The listing builds one solid part. Answer for the finished solid, in the listing's coordinates (mm). Round coordinates to 2 decimals unless told otherwise and drop trailing zeros. Write each loop counter-clockwise with the first axis right and the second up, starting at its lowest first coordinate (ties: lowest second). Pieces come first, ordered by that corner, then holes.
Autodesk Inventor part; units mm, degrees
ref_plane "YZ Plane" through (0, 0, 0) normal (1, 0, 0) x (0, 1, 0)
ref_plane "XZ Plane" through (0, 0, 0) normal (0, 1, 0) x (-1, 0, 0)
ref_plane "XY Plane" through (0, 0, 0) normal (0, 0, 1) x (1, 0, 0)
sketch "Sketch1" plane through (0, 0, 0) normal (0, 1, 0) x (-1, 0, 0)
  arc A0 (0, -273.05) -> (273.05, 0) centre (0, 0) ccw
  arc A1 (0, -285.75) -> (285.75, 0) centre (0, 0) ccw
  arc A2 (0, -146.05) -> (146.05, 0) centre (0, 0) ccw
  arc A3 (0, -133.35) -> (133.35, 0) centre (0, 0) ccw
  line L0 (0, -285.75) -> (-6.35, -285.75)
  line L1 (146.05, 0) -> (146.05, 6.35)
  line L2 (133.35, 0) -> (133.35, 6.35)
  line L3 (273.05, 6.35) -> (273.05, 0)
  line L4 (285.75, 6.35) -> (285.75, 0)
  circle A4 centre (103.1708, -94.1906) radius 3.3782
  circle A5 centre (94.1906, -103.1708) radius 3.3782
  circle A6 centre (279.4, 0) radius 3.3782
  circle A7 centre (139.7, 0) radius 3.3782
  circle A8 centre (202.0047, -193.0245) radius 3.3782
  circle A9 centre (193.0245, -202.0047) radius 3.3782
  circle A10 centre (0, -279.4) radius 3.3782
  circle A11 centre (0, -139.7) radius 3.3782
  circle A12 centre (-55.2746, -139.7) radius 3.3782
  circle A13 centre (-78.3684, -279.4) radius 3.3782
  line L5 (285.75, 6.35) -> (273.05, 6.35)
  line L6 (146.05, 6.35) -> (133.35, 6.35)
  line L7 (-314.96, -285.75) -> (-314.96, -273.05)
  line L8 (-101.6, -133.35) -> (-127, -133.35)
  line L9 (-127, -146.05) -> (-101.6, -146.05)
  line L10 (-314.96, -146.05) -> (-314.96, -133.35)
  line L11 (-6.35, -285.75) -> (-6.35, -393.7)
  line L12 (-6.35, -393.7) -> (-314.325, -393.7)
  line L13 (-314.325, -393.7) -> (-314.325, -76.2)
  line L14 (-314.325, -76.2) -> (-120.65, -76.2)
  line L15 (-120.65, -76.2) -> (0, -133.35)
  line L16 (0, -285.75) -> (-6.35, -285.75)
  line L17 (0, -146.05) -> (0, -273.05)
  dimension "d10" = 12.7
  dimension "d11" = 12.7
  dimension "d13" = 12.7
  dimension "d14" = 6.7564
  dimension "d15" = 6.7564
  dimension "d16" = 6.7564
  dimension "d18" = 6.7564
  dimension "d20" = 6.35
  dimension "d21" = 6.7564
  dimension "d22" = 6.7564
  dimension "d23" = 6.7564
  dimension "d26" = 6.7564
  dimension "d30" = 6.7564
  dimension "d32" = 6.7564
  dimension "d66" = 25.4
  dimension "d67" = 0
  dimension "d72" = 12.7
  dimension "d81" = 107.95
  dimension "d82" = 133.35
  dimension "d83" = 279.4
  dimension "d84" = 6.35
  dimension "d85" = 317.5
  dimension "d86" = 193.675
  dimension "d87" = 55.2746
  dimension "d88" = 139.7
  dimension "d91" = 307.975
extrude "Extrusion7" add sketch "Sketch1" along normal blind 6.35
sketch "Sketch7" plane through (0, 0, 0) normal (0, -1, 0) x (1, 0, 0)
  line L0 (0, -273.05) -> (0, -146.05)
  line L1 (314.325, -76.2) -> (314.325, -393.7)
  line L2 (314.325, -234.95) -> (0, -234.95)
  line L3 (301.625, -139.7) -> (301.625, -165.1)
  line L4 (301.625, -165.1) -> (98.425, -165.1)
  line L5 (98.425, -165.1) -> (98.425, -139.7)
  line L6 (98.425, -139.7) -> (301.625, -139.7)
  line L7 (301.625, -330.2) -> (301.625, -304.8)
  line L8 (301.625, -304.8) -> (98.425, -304.8)
  line L9 (98.425, -304.8) -> (98.425, -330.2)
  line L10 (98.425, -330.2) -> (301.625, -330.2)
  dimension "d92" = 25.4
  dimension "d93" = 203.2
  dimension "d94" = 12.7
  dimension "d95" = 69.85
extrude "Extrusion8" cut sketch "Sketch7" against normal blind 6.35
sketch "Sketch8" plane through (0, 6.35, 0) normal (0, 1, 0) x (1, 0, 0)
  line L0 (98.425, 165.1) -> (301.625, 165.1)
  line L1 (301.625, 304.8) -> (98.425, 304.8)
  circle A0 centre (78.3684, 279.4) radius 3.3782
  line L2 (314.325, 76.2) -> (314.325, 393.7)
  line L3 (314.325, 393.7) -> (6.35, 393.7)
  line L4 (0, 273.05) -> (0, 146.05)
  line L5 (295.275, 367.3082) -> (295.275, 342.9)
  line L6 (295.275, 342.9) -> (28.575, 342.9)
  line L7 (28.575, 342.9) -> (28.575, 371.475)
  line L8 (28.575, 371.475) -> (295.275, 371.475)
  line L9 (295.275, 371.475) -> (295.275, 367.3082)
  line L10 (295.275, 292.1) -> (28.575, 292.1)
  line L11 (28.575, 292.1) -> (28.575, 263.525)
  line L12 (28.575, 263.525) -> (295.275, 263.525)
  line L13 (295.275, 263.525) -> (295.275, 292.1)
  line L14 (295.275, 250.825) -> (28.575, 250.825)
  line L15 (28.575, 250.825) -> (28.575, 222.25)
  line L16 (28.575, 222.25) -> (295.275, 222.25)
  line L17 (295.275, 222.25) -> (295.275, 250.825)
  line L18 (295.275, 209.55) -> (295.275, 180.975)
  line L19 (295.275, 180.975) -> (28.575, 180.975)
  line L20 (28.575, 180.975) -> (28.575, 209.55)
  line L21 (28.575, 209.55) -> (295.275, 209.55)
  dimension "d100" = 90
  dimension "d101" = 22.225
  dimension "d102" = 19.05
  dimension "d103" = 28.575
  dimension "d104" = 266.7
  dimension "d105" = 28.575
  dimension "d106" = 19.05
  dimension "d107" = 12.7
  dimension "d108" = 266.7
  dimension "d109" = 28.575
  dimension "d110" = 28.575
  dimension "d111" = 12.7
  dimension "d112" = 12.7
  dimension "d113" = 266.7
  dimension "d114" = 19.05
  dimension "d115" = 19.05
extrude "Extrusion9" cut sketch "Sketch8" against normal blind 25.4
sketch "Sketch9" plane through (0, 6.35, 0) normal (0, 1, 0) x (1, 0, 0)
  line L0 (314.325, 76.2) -> (314.325, 393.7)
  line L1 (295.275, 371.475) -> (295.275, 88.9)
  line L2 (295.275, 88.9) -> (288.925, 88.9)
  line L3 (288.925, 88.9) -> (288.925, 381)
  line L4 (288.925, 381) -> (295.275, 381)
  line L5 (295.275, 381) -> (295.275, 371.475)
  dimension "d118" = 282.575
  dimension "d119" = 6.35
  dimension "d120" = 292.1
extrude "Extrusion10" cut sketch "Sketch9" against normal blind 25.4
sketch "Sketch10" plane through (0, 6.35, 0) normal (0, 1, 0) x (1, 0, 0)
  line L0 (120.65, 76.2) -> (314.325, 76.2)
  line L1 (0, 273.05) -> (0, 146.05)
  line L2 (120.65, 76.2) -> (120.65, 63.5)
  line L3 (120.65, 63.5) -> (145.3457, 38.8043)
  line L4 (145.3457, 38.8043) -> (302.8387, 38.8043)
  line L5 (302.8387, 38.8043) -> (302.8387, 76.2)
  dimension "d123" = 12.7
  dimension "d124" = 34.925
  dimension "d125" = 135
extrude "Extrusion11" add sketch "Sketch10" against normal blind 6.35
sketch "Sketch13" plane through (0, 6.35, 0) normal (0, 1, 0) x (1, 0, 0)
  line L0 (288.925, 88.9) -> (288.925, 139.7)
  line L1 (288.925, 139.7) -> (98.425, 139.7)
  line L2 (288.925, 381) -> (295.275, 381)
  line L3 (295.275, 88.9) -> (288.925, 88.9)
  line L4 (145.3457, 38.8043) -> (302.8387, 38.8043)
  line L5 (302.8387, 38.8043) -> (302.8387, 76.2)
  line L6 (0, 273.05) -> (0, 146.05)
  line L7 (98.425, 127) -> (98.425, 101.6)
  line L8 (98.425, 101.6) -> (288.925, 101.6)
  line L9 (98.425, 127) -> (288.925, 127)
  line L10 (288.925, 88.9) -> (288.925, 44.45)
  line L11 (288.925, 44.45) -> (295.275, 44.45)
  line L12 (295.275, 44.45) -> (295.275, 88.9)
  dimension "d135" = 25.4
  dimension "d136" = 336.55
  dimension "d137" = 12.7
extrude "Extrusion13" cut sketch "Sketch13" against normal blind 25.4
sketch "Sketch14" plane through (0, 6.35, 0) normal (0, 1, 0) x (1, 0, 0)
  line L0 (311.15, 79.375) -> (304.8, 79.375)
  line L1 (304.8, 79.375) -> (304.8, 85.725)
  line L2 (304.8, 85.725) -> (311.15, 85.725)
  line L3 (311.15, 85.725) -> (311.15, 79.375)
  line L4 (6.35, 381) -> (301.625, 381)
  line L5 (301.625, 381) -> (301.625, 76.2)
  line L6 (301.625, 76.2) -> (314.325, 76.2)
  line L7 (314.325, 76.2) -> (314.325, 393.7)
  line L8 (314.325, 393.7) -> (6.35, 393.7)
  line L9 (6.35, 393.7) -> (6.35, 381)
  line L10 (311.15, 390.525) -> (311.15, 384.175)
  line L11 (311.15, 384.175) -> (304.8, 384.175)
  line L12 (304.8, 384.175) -> (304.8, 390.525)
  line L13 (304.8, 390.525) -> (311.15, 390.525)
  line L14 (15.875, 384.175) -> (9.525, 384.175)
  line L15 (9.525, 384.175) -> (9.525, 390.525)
  line L16 (9.525, 390.525) -> (15.875, 390.525)
  line L17 (15.875, 390.525) -> (15.875, 384.175)
  line L18 (145.3457, 38.8043) -> (302.8387, 38.8043)
  line L19 (301.625, 139.7) -> (295.275, 139.7)
  line L20 (152.2186, 54.6793) -> (152.2186, 48.3293)
  line L21 (152.2186, 48.3293) -> (158.5686, 48.3293)
  line L22 (158.5686, 48.3293) -> (158.5686, 54.6793)
  line L23 (158.5686, 54.6793) -> (152.2186, 54.6793)
  dimension "d146" = 6.35
  dimension "d148" = 6.35
  dimension "d149" = 9.525
extrude "Extrusion15" cut sketch "Sketch14" against normal blind 25.4 contours L23 L22 L21 L20
sketch "Sketch16" plane through (0, 6.35, 0) normal (0, 1, 0) x (1, 0, 0)
  line L0 (288.925, 165.1) -> (288.925, 180.975)
  line L1 (288.925, 209.55) -> (288.925, 222.25)
  line L2 (288.925, 250.825) -> (288.925, 263.525)
  line L3 (288.925, 292.1) -> (288.925, 304.8)
  line L4 (295.275, 304.8) -> (295.275, 165.1)
  line L5 (295.275, 165.1) -> (301.625, 165.1)
  line L6 (288.925, 165.1) -> (295.275, 165.1)
  line L7 (288.925, 180.975) -> (295.275, 180.975)
  line L8 (288.925, 222.25) -> (295.275, 222.25)
  line L9 (288.925, 209.55) -> (295.275, 209.55)
  line L10 (288.925, 304.8) -> (295.275, 304.8)
  line L11 (288.925, 292.1) -> (295.275, 292.1)
  line L12 (288.925, 263.525) -> (295.275, 263.525)
  line L13 (288.925, 250.825) -> (295.275, 250.825)
extrude "Extrusion16" add sketch "Sketch16" against normal blind 6.35
sketch "Sketch17" plane through (0, 6.35, 0) normal (0, 1, 0) x (1, 0, 0)
  line L0 (288.925, 44.45) -> (288.925, 101.6)
  line L1 (288.925, 101.6) -> (98.425, 101.6)
  line L2 (98.425, 127) -> (288.925, 127)
  line L3 (288.925, 342.9) -> (28.575, 342.9)
  line L4 (28.575, 371.475) -> (288.925, 371.475)
  line L5 (288.925, 127) -> (288.925, 101.6)
  line L6 (276.225, 127) -> (276.225, 101.6)
  line L7 (288.925, 342.9) -> (288.925, 371.475)
  line L8 (276.225, 371.475) -> (276.225, 342.9)
  dimension "d155" = 12.7
  dimension "d156" = 12.7
extrude "Extrusion17" add sketch "Sketch17" against normal blind 6.35
sketch "Sketch18" plane through (0, 6.35, 0) normal (0, 1, 0) x (1, 0, 0)
  line L0 (288.925, 44.45) -> (288.925, 139.7)
  line L1 (295.275, 139.7) -> (295.275, 44.45)
  line L2 (295.275, 44.45) -> (288.925, 44.45)
  line L3 (145.3457, 38.8043) -> (302.8387, 38.8043)
  line L4 (295.275, 70.5543) -> (288.925, 70.5543)
  dimension "d159" = 31.75
extrude "Extrusion18" add sketch "Sketch18" against normal blind 6.35
sketch "Sketch19" plane through (0, 6.35, 0) normal (0, 1, 0) x (1, 0, 0)
  line L0 (314.325, 393.7) -> (6.35, 393.7)
  line L1 (6.35, 393.7) -> (6.35, 285.75)
  circle A0 centre (76.2, 387.35) radius 3.3782
  dimension "d162" = 6.7564
  dimension "d164" = 6.35
  dimension "d165" = 69.85
extrude "Extrusion19" cut sketch "Sketch19" against normal blind 25.4
sketch "Sketch20" plane through (0, 6.35, 0) normal (0, 1, 0) x (1, 0, 0)
  circle A0 centre (95.25, 387.35) radius 3.3782
extrude "Extrusion20" cut sketch "Sketch20" against normal blind 25.4
sketch "Sketch21" plane through (0, 6.35, 0) normal (0, 1, 0) x (1, 0, 0)
  line L0 (158.5686, 54.6793) -> (158.5686, 48.3293)
  line L1 (145.3457, 38.8043) -> (302.8387, 38.8043)
  line L2 (302.8387, 38.8043) -> (302.8387, 76.2)
  circle A0 centre (155.3936, 67.3793) radius 3.3782
  circle A1 centre (267.9137, 67.3793) radius 3.3782
  dimension "d170" = 6.7564
  dimension "d171" = 6.7564
  dimension "d172" = 28.575
  dimension "d173" = 34.925
  dimension "d174" = 28.575
  dimension "d176" = 3.175
extrude "Extrusion21" cut sketch "Sketch21" against normal blind 25.4
sketch "Sketch22" plane through (0, 6.35, 0) normal (0, 1, 0) x (1, 0, 0)
  line L0 (288.925, 330.2) -> (288.925, 381)
  line L1 (288.925, 381) -> (295.275, 381)
  line L2 (295.275, 381) -> (295.275, 330.2)
  line L3 (288.925, 358.775) -> (295.275, 358.775)
  dimension "d179" = 22.225
extrude "Extrusion22" add sketch "Sketch22" against normal blind 6.35
sketch "Sketch23" plane through (0, 6.35, 0) normal (0, 1, 0) x (1, 0, 0)
  line L0 (158.5686, 48.3293) -> (152.2186, 48.3293)
  line L1 (152.2186, 48.3293) -> (152.2186, 54.6793)
  line L2 (152.2186, 54.6793) -> (158.5686, 54.6793)
  line L3 (158.5686, 54.6793) -> (158.5686, 48.3293)
  line L4 (120.65, 63.5) -> (145.3457, 38.8043)
  line L5 (145.3457, 38.8043) -> (302.8387, 38.8043)
  line L6 (302.8387, 38.8043) -> (302.8387, 76.2)
  line L7 (28.575, 371.475) -> (276.225, 371.475)
  line L8 (302.8387, 61.0293) -> (123.1207, 61.0293)
  dimension "d182" = 22.225
extrude "Extrusion23" cut sketch "Sketch23" against normal blind 6.35
sketch "Sketch24" plane through (0, 6.35, 0) normal (0, 1, 0) x (1, 0, 0)
  line L0 (276.225, 127) -> (276.225, 101.6)
  line L1 (276.225, 101.6) -> (98.425, 101.6)
  line L2 (98.425, 101.6) -> (98.425, 127)
  line L3 (98.425, 127) -> (276.225, 127)
extrude "Extrusion24" add sketch "Sketch24" against normal blind 6.35
sketch "Sketch25" plane through (0, 6.35, 0) normal (0, 1, 0) x (1, 0, 0)
  line L0 (295.275, 222.25) -> (28.575, 222.25)
  line L1 (295.275, 209.55) -> (295.275, 180.975)
  line L2 (28.575, 209.55) -> (295.275, 209.55)
  line L3 (295.275, 70.5543) -> (288.925, 70.5543)
  line L4 (28.575, 209.55) -> (28.575, 222.25)
  line L5 (295.275, 222.25) -> (295.275, 209.55)
extrude "Extrusion25" cut sketch "Sketch25" against normal blind 25.4
properties part number "Runner Rails v2" material "Polycarbonate, Clear"
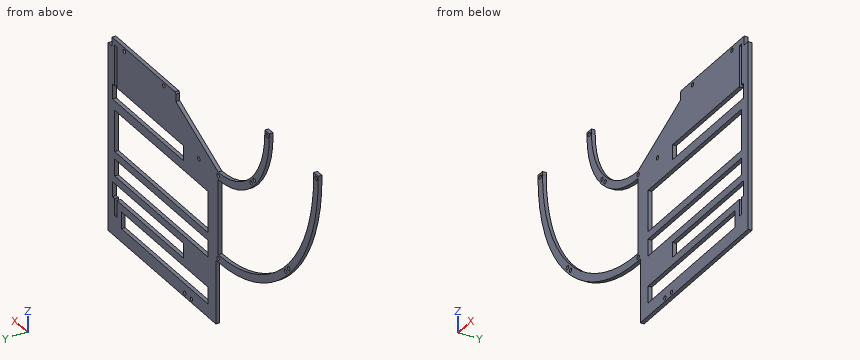
1. Given pin 1 (3 mm diameter, centred on x = 193, y = 1.5, fed in from +Z); pin 2 (1.9 mm diameter, centred on y = 3, z = -359, fed in from -X); pin 3 (10 mm diameter, centred on x = 152, z = -159, fed in from -Y); pin 4 (11 mm diameter, centred on x = -279.4, z = 0, fed in from -Y), each flat-ended and moving along its own axis, determine where each tip first touches the part or whether it passes through.
Geometry says:
pin 1: stops at z = -61.03
pin 2: stops at x = 6.35
pin 3: passes through
pin 4: stops at y = 0
2. Section D-D on x = 66 is taken. Determine the outline of the cut face in (y, z) (3 decimals).
Geometry says:
outline: (0, -393.7) - (6.35, -393.7) - (6.35, -371.475) - (0, -371.475) - close; (0, -342.9) - (6.35, -342.9) - (6.35, -292.1) - (0, -292.1) - close; (0, -263.525) - (6.35, -263.525) - (6.35, -250.825) - (0, -250.825) - close; (0, -180.975) - (6.35, -180.975) - (6.35, -102.087) - (0, -102.087) - close
3. Section A-A on x = 251 is taken. Determine the outline of the cut face in (y, z) (3 decimals).
Geometry says:
outline: (0, -393.7) - (6.35, -393.7) - (6.35, -371.475) - (0, -371.475) - close; (0, -342.9) - (6.35, -342.9) - (6.35, -330.2) - (0, -330.2) - close; (0, -304.8) - (6.35, -304.8) - (6.35, -292.1) - (0, -292.1) - close; (0, -263.525) - (6.35, -263.525) - (6.35, -250.825) - (0, -250.825) - close; (0, -180.975) - (6.35, -180.975) - (6.35, -165.1) - (0, -165.1) - close; (0, -139.7) - (6.35, -139.7) - (6.35, -61.029) - (0, -61.029) - close
4. Section C-C on y = 2.25 is taken. Give the number of separate pieces and of enclosed holes in the cut face, plus the area to 3 significant figures.
Geometry says:
separate pieces: 1
enclosed holes: 18
area: 62,200 mm2
5. Straight lines are drawn through the part: line 1 along Z through (x, y) = (217.5, 3) (3 decimals); line 2 along Z through (x, y) = (285, 4.5) (3 decimals); line 3 along X through (y, z) = (5, -349) (3 decimals). For each, find the intervals that lie inside material, in ascending order.
Geometry says:
line 1: z = -393.7 to -371.475, -342.9 to -330.2, -304.8 to -292.1, -263.525 to -250.825, -180.975 to -165.1, -139.7 to -61.029
line 2: z = -393.7 to -330.2, -304.8 to -292.1, -263.525 to -250.825, -180.975 to -165.1, -139.7 to -61.029
line 3: x = 6.35 to 28.575, 276.225 to 288.925, 295.275 to 314.325
6. Section B-B on x = -28 is taken. Determine the outline of the cut face in (y, z), plus the area to 3 significant figures.
Geometry says:
outline: (0, -284.37) - (6.35, -284.37) - (6.35, -271.61) - (0, -271.61) - close; (0, -143.34) - (6.35, -143.34) - (6.35, -130.38) - (0, -130.38) - close
area: 163 mm2
